Autodesk Inventor part; units mm, degrees
ref_plane "YZ Plane" through (0, 0, 0) normal (1, 0, 0) x (0, 1, 0)
ref_plane "XZ Plane" through (0, 0, 0) normal (0, 1, 0) x (-1, 0, 0)
ref_plane "XY Plane" through (0, 0, 0) normal (0, 0, 1) x (1, 0, 0)
sketch "Sketch1" plane through (0, 0, 0) normal (0, 1, 0) x (-1, 0, 0)
  line L0 (-4.5709, 0.1557) -> (-12.5709, 0.1557)
  line L1 (-12.5709, 0.1557) -> (-12.5709, 1.3557)
  line L2 (-12.5709, 1.3557) -> (-4.5709, 1.3557)
  line L3 (-4.5709, 1.3557) -> (-4.5709, 0.1557)
  dimension "d27" = 8
  dimension "d28" = 1.2
extrude "Plate4" add sketch "Sketch1" along normal blind 0.25
sketch "Sketch5" plane through (12.3209, 0.25, 1.3557) normal (1, 0, 0) x (0, 1, 0)
  line L0 (0, -1.2) -> (0, 0)
  line L1 (0, 0) -> (-5.7, 0)
  line L2 (-5.7, 0) -> (-5.7, -1.2)
  line L3 (-5.7, -1.2) -> (0, -1.2)
edge flange "Flange4" height 5.7 angle 90 thickness 0.25 bend radius 0.25 thickness toward (1, 0, 0) relief tear relief width 0.25 relief depth 0.125 corner gap 0.25 corner form 0 edges at (12.5709, 0, 0.7557) (4.5709, 0, 0.7557) wall of the first edge with corners at (12.3209, 0.25, 0.1557) (12.3209, 0.25, 1.3557) (12.3209, -5.45, 1.3557) (12.3209, -5.45, 0.1557)
bend "Bend4"
corner "Corner4"
sketch "Sketch6" plane through (12.5709, -5.45, 1.3557) normal (1, 0, 0) x (0, 0, -1)
  line L0 (1.2, 0) -> (0, 0)
  line L1 (0.6, 0) -> (0.6, 5.2) construction
  line L2 (1.2, 5.2) -> (0, 5.2)
  line L3 (1.2, 3.4021) -> (0.85, 3.2)
  line L4 (0.85, 3.2) -> (0.85, 0)
  line L5 (1.2, 0) -> (0.85, 0)
  line L6 (1.2, 5.2) -> (1.2, 0)
  line L7 (1.2, 3.4021) -> (1.2, 0)
  line L8 (0, 5.7) -> (1.2, 5.7)
  point P0 (1.3557, 5.45)
  dimension "d52" = 3.2
  dimension "d54" = 0.25
  dimension "d56" = 2.5
extrude "Cut1" cut sketch "Sketch6" against normal blind 0.25
ref_plane "Work Plane1" through (12.5709, -0.25, 0.7557) normal (0, 0, -1) x (-1, 0, 0)
ref_plane "Work Plane2" through (8.5709, -5.45, 1.3557) normal (1, 0, 0) x (0, 0, -1)
mirror "Mirror2" about plane through (8.5709, -5.45, 1.3557) normal (1, 0, 0) of "Cut1"
sketch "Sketch7" plane through (8.5709, -5.45, 1.3557) normal (1, 0, 0) x (0, 0, -1)
  line L0 (0, 0) -> (0.85, 0)
  line L1 (0, 5.7) -> (1.2, 5.7)
  line L2 (0, 0) -> (0.35, 0)
  line L3 (0.35, 0) -> (0.35, 5.7)
  line L4 (0.35, 5.7) -> (0, 5.7)
  line L5 (0, 5.7) -> (0, 0)
  line L6 (1.2, 5.7) -> (1.2, 5.45)
  line L7 (1.2, 5.45) -> (0, 5.45)
  line L8 (0, 5.45) -> (0, 5.7)
  line L9 (0, 5.7) -> (1.2, 5.7)
  line L10 (0.6, 6.84) -> (0.6, -1.14)
  point P0 (1.3557, 5.45)
  dimension "d57" = 0.25
extrude "Cut2" cut sketch "Sketch7" along normal through all both and the other way through all contours L5 L7 L3 L0 | L5 L1 L3 L7
equation "\"d27\" = atmegaPinBaseWidth"
equation "\"d28\" = atmegaPinWidth1"
equation "\"d52\" = atmegaSeatingPlaneDistance"
equation "\"d54\" = 0.5 * atmegaPinWidth2"
equation "\"d50\" = Thickness"
equation "\"d57\" = 0.5 * atmegaPinWidth2"
equation "\"d58\" = Thickness"
equation "\"d29\" = Thickness"
equation "\"d40\" = BendReliefWidth"
equation "\"d41\" = BendReliefDepth"
equation "\"d42\" = MinimumRemnant"
equation "\"d43\" = TransitionRadius"
equation "\"d44\" = atmegaPinLenght"
equation "\"d46\" = BendRadius"
equation "\"d47\" = CornerReliefSize"
equation "\"d48\" = GapSize"
equation "\"d49\" = JacobiRadiusSize"
equation "\"BendRadius\" = Thickness"
equation "\"BendReliefWidth\" = Thickness"
equation "\"BendReliefDepth\" = 0.5 * Thickness"
equation "\"CornerReliefSize\" = 4 * Thickness"
equation "\"MinimumRemnant\" = 2 * Thickness"
equation "\"TransitionRadius\" = BendRadius"
equation "\"JacobiRadiusSize\" = BendRadius"
equation "\"GapSize\" = Thickness"
equation "\"atmegaPinThickness\" = 0.3"
equation "\"atmegaPinWidth1\" = 1.2"
equation "\"atmegaPinWidth2\" = 0.5"
equation "\"atmegaEndPinWidth\" = 0.9"
equation "\"atmegaPinBendAngle\" = 80deg"
equation "\"atmegaPinBaseWidth\" = 8"
equation "\"atmegaSeatingPlaneDistance\" = 3.2"
properties part number "atmega_pin"
The model under review builds one solid part; all positions refer to its coordinate system, in mm. A direction names the side the tool comes from. Give positions to 0.01 mm unless a question says otherwise; leave off trailing zeros. Order: outer loops, then holes, each group sorted by start corner. A loop starts at its lowest first (then second) coordinate and runs counter-clockwise, first axis right, second up. Notation, with made-up numbers: (67.5, -32.75) - (111.5, -32.75) arc R10 cw to (111.5, -15.75) - close; hole circle Ø1 at (25.5, -10). An arc over 180 degrees is marked (long way). Use CSV: the item, a comma, the result in double quotes. Start each with the question number.
Q1. We need section D-D, the plane x = 5.5. Write out the cut boundary in (y, z).
Q2. We need section A-A, the plane y = -2.7. Write out the cut boundary in (x, z).
Q3. To check wall thickness, follow line 1 along X through (y, z) = (-0.6, 0.9); line 2 along Y through (x, z) = (12, 0.7). State the ranges of each line that lie inside material, in increasing order. Write a range as [from, to].
Q4. We need section B-B, the plane z = 0.9. Write out the cut boundary in (x, y), and give its area (3 significant figures).
Q5. The part is to be moulded in two halves that separate along X. For faces 3 (the flat face through (12.571, -2.3, 0.7)), 4 (the flat face through (4.821, -2.2, 0.7)), 5 (the flat face through (8.6, 0.25, 0.6)), say which applies: +X half, -X half, draft (parallel to the pull), parting line (faces both ways), or undercut.
Q6. Tool access review of faces 1 (the flat face through (8.6, 0, 0.6)), 2 (the flat face through (4.571, -2.3, 0.7)): name each direction out of +Z, -Z, +X, -X, +Y, -Y from which nothing blocks a thin tool from reaching the whole face with its end or side.
Q7. We need section C-C, the plane y = -0.5. Write out the cut boundary in (x, z), and give its area (3 significant figures).
Outcome:
1,outline,"(0, 0.16) - (0.25, 0.16) - (0.25, 1.01) - (0, 1.01) - close"
2,outline,"(4.57, 0.51) - (4.82, 0.51) - (4.82, 1.01) - (4.57, 1.01) - close; (12.32, 0.51) - (12.57, 0.51) - (12.57, 1.01) - (12.32, 1.01) - close"
3,line 1,"x = [4.57, 4.82], [12.32, 12.57]"
3,line 2,"y = [0, 0.25]"
4,outline,"(4.57, -5.45) - (4.82, -5.45) - (4.82, -0.25) arc R0.25 cw to (5.07, 0) - (12.07, 0) arc R0.25 cw to (12.32, -0.25) - (12.32, -5.45) - (12.57, -5.45) - (12.57, -0.25) arc R0.5 ccw to (12.07, 0.25) - (5.07, 0.25) arc R0.5 ccw to (4.57, -0.25) - close"
4,area,"4.64 mm^2"
5,face 3,"+X half"
5,face 4,"undercut"
5,face 5,"draft"
6,face 1,"+Z, -Z, -Y"
6,face 2,"+Z, -Z, -X, +Y, -Y"
7,outline,"(4.57, 0.16) - (4.82, 0.16) - (4.82, 1.01) - (4.57, 1.01) - close; (12.32, 0.16) - (12.57, 0.16) - (12.57, 1.01) - (12.32, 1.01) - close"
7,area,"0.425 mm^2"
